```python
from build123d import *

# Parameters (mm, degrees)
BOX001_W                  = 500
BOX001_H                  = 500
BOX001_DEPTH              = 500
BOX001_PLACEMENT_ANGLE    = 2
TUBE034_R                 = 85
TUBE034_R_2               = 80
TUBE034_DEPTH             = 21
TUBE033_R                 = 100
TUBE033_R_2               = 80
TUBE033_DEPTH             = 200
PAD032_DEPTH              = 100
PAD033_DEPTH              = 2
COMMON014_PLACEMENT_ANGLE = 45
ARRAY014_COUNT            = 22
ARRAY014_PLACEMENT_ANGLE  = 180
TUBE035_R                 = 34
TUBE035_R_2               = 30
TUBE035_DEPTH             = 21


with BuildPart() as cube001:
    # Box001 → Box001 (new body)
    with BuildSketch(Plane.XY):
        with Locations((250, 250)):
            Rectangle(BOX001_W, BOX001_H)
    extrude(amount=BOX001_DEPTH)


with BuildPart() as cube001_1:
    # Box001 placement: moved
    add(cube001.part.moved(Location((8.73, -250, 0))).rotate(Axis((8.73, -250, 0), (0, 0, 1)), BOX001_PLACEMENT_ANGLE))


with BuildPart() as tube034:
    # Tube034 → Tube034 (new body)
    with BuildSketch(Plane.XY.offset(139.5)):
        Circle(TUBE034_R)
        Circle(TUBE034_R_2, mode=Mode.SUBTRACT)
    extrude(amount=TUBE034_DEPTH)


with BuildPart() as tube033:
    # Tube033 → Tube033 (new body)
    with BuildSketch(Plane.XY):
        Circle(TUBE033_R)
        Circle(TUBE033_R_2, mode=Mode.SUBTRACT)
    extrude(amount=TUBE033_DEPTH)


with BuildPart() as body033:
    # Sketch032 → Pad032 (new body)
    with BuildSketch(Plane.XZ):
        Polygon((0, 0), (0, 2), (26, 0.9), (26, 0), align=None)
    extrude(amount=PAD032_DEPTH)


with BuildPart() as body033_1:
    # Body033 placement: moved
    add(body033.part.moved(Location((-5, 0, 5))))


with BuildPart() as cut008:
    # Sketch033 → Pad033 (new body)
    with BuildSketch(Plane.XY):
        Polygon((0, 0), (0, -52), (25.94305, -47.924315), (8.5, 0), align=None)
    extrude(amount=PAD033_DEPTH)


with BuildPart() as cut008_1:
    # Body034 placement: moved
    add(cut008.part.moved(Location((-5, -33, 5))))

    # Common014: intersect Body033
    add(body033_1.part, mode=Mode.INTERSECT)


with BuildPart() as cut008_2:
    # Common014 placement: moved
    add(cut008_1.part.rotate(Axis((0, 0, 0), (0, 1, 0)), COMMON014_PLACEMENT_ANGLE))

    # Array014: Cut008 ×22 about axis
    array014_axis = Axis((0, 0, 0), (0, 0, 1))


with BuildPart() as cut008_3:
    add(cut008_2.part)
    for i in range(1, ARRAY014_COUNT):
        add(cut008_2.part.rotate(array014_axis, i * 360 / ARRAY014_COUNT))


with BuildPart() as cut008_4:
    # Array014 placement: moved
    add(cut008_3.part.moved(Location((0, 0, 149))).rotate(Axis((0, 0, 149), (0, 1, 0)), ARRAY014_PLACEMENT_ANGLE))

    # Cut008: cut Tube033
    add(tube033.part, mode=Mode.SUBTRACT)


with BuildPart() as obj1:
    # Tube035 → Tube035 (new body)
    with BuildSketch(Plane.XY.offset(139.5)):
        Circle(TUBE035_R)
        Circle(TUBE035_R_2, mode=Mode.SUBTRACT)
    extrude(amount=TUBE035_DEPTH)

    # Fusion016: union Tube034, Cut008
    add(tube034.part)
    add(cut008_4.part)

    # Cut009: cut Cube001
    add(cube001_1.part, mode=Mode.SUBTRACT)


solid = obj1.part
```
Verification items for the finished model (mm, model axes). A direction names the side the tool comes from. Give positions to 0.01 mm unless a question says otherwise; leave off trailing zeros. Put each result on its own line as item: value.
Q1. Scan lines: probe 1 along X at (y, z) = (-65, 144.5); probe 2 along X at (y, z) = (31, 140.75); probe 3 along Y at (x, z) = (-41.5, 154.75). Record each from-to range of solid material in increasing order. Write a range as from..to.
Result:
probe 1: -54.77..-44.83, -24.38..-21.77, -5.08..-2.57
probe 2: -79.15..-73.75, -65.04..-63.96, -33.98..-33.29, -18.52..-17.98, -13.96..-1.08
probe 3: -74.18..-68.39, 52.92..55.14, 68.39..74.18
Q2. Depth check by flat-ended pin: P1, Ø3, axis at y = 9.5, z = 156, coming from the -X side; P2, Ø2, axis at y = 46, z = 151, coming from the -X side; P3, Ø6, axis at x = -35, z = 152, coming from the -Y side. Enter the tip coordinate at first touch or a pass-through.
Result:
P1: x = -84.62
P2: x = -72.11
P3: y = -78.75
Q3. Set-up check for faces 1 (the face through (-31, 0, 160.5)), 2 (the face through (-3.9, 57.16, 153.4)), 3 (the face through (-41.326, 46.181, 147.506)), 4 (the face through (-38.94, -48.16, 148.65)): record each of +Z, -Z, +X, -X, +Y, -Y from which the full face is reachable in a straight line by a thin tool's end or side.
Result:
face 1: +Z, +X, -X, +Y, -Y
face 2: +Z, +X
face 3: -Z
face 4: +Z
